Input: part model. Units: mm. Frame: model coordinates. A direction names the side the tool comes from. Round coordinates to 2 decimals unless told otherwise and drop trailing zeros. Loops run counter-clockwise (first coordinate to the right, second up) from the corner with the lowest first, then second, coordinate; pieces in that order, holes last. Notation, with made-up numbers: M 69,44 L 105,44 A26 ccw 105,69 Z; hole C 74.25,5.5 d11. An arc over 180 degrees is marked long. Use one line per item in the form item = value. Start each with the question number.
Q1. Section query B-B, the plane x = 4.5. Output: boundary loops of the cut face in (y, z), and give its area (3 significant figures).
Q2. Ray query, line 1 along Z through (x, y) = (-3, 0.65); line 2 along Z through (x, y) = (13.5, 1); line 3 along X through (y, z) = (0.8, 5.75). Return the intervals inside material, ascending.
Q3. Section query A-A, the plane z = -3. Output: boundary loops of the cut face in (x, y), and give its area (3 significant figures).
Q4. First-contact query: P1, Ø0.9, axis at x = 17.5, y = 0, coming from the +Z side; P2, Ø0.9, axis at x = 17, y = -1, coming from the -Z side. Flat tips, straight axial feed; report the tip coordinate or a pass-through.
Q5. Section query D-D, the plane z = 0. Output: boundary loops of the cut face in (x, y), and give its area (3 significant figures).
Q6. Mould query, pull axis Z, two halves, no side actions, for faces 4 (the flat face through (0, -2.5, 11)), 5 (the cylindrical face through (17.64, -0.04, -11.1)), 6 (the cylindrical face through (-12.64, -0.04, -8.1)). Classes: pulls with the +Z half, pulls with the -Z half, needs draft (parallel to the pull), parting line crosses it, or undercut.
Q7. Section query C-C, the plane y = 1.5. Output: boundary loops of the cut face in (x, z), and give its area (3 significant figures).
Q8. Access query for faces 1 (the flat face through (17, 0, -2)), 2 (the flat face through (1, 0, 9)), 3 (the flat face through (0, 2.5, 11)). Directions: +Z, -Z, +X, -X, +Y, -Y. A direction counts if a zero-diameter tool reaches every point of the face in a straight line with its end or side. Return the directions, or none.
```python
from build123d import *

# Parameters (mm, degrees)
F1_DEPTH = 2.5
F2_R     = 3


with BuildPart() as f1:
    # F0 (on Front) → F1 (new body, symmetric)
    with BuildSketch(Plane.XZ):
        with BuildLine():
            Line((18.5, 12), (-18.5, 12))
            Line((-18.5, 12), (-18.5, -12))
            Line((-18.5, -12), (18.5, -12))
            Line((18.5, -12), (18.5, -2))
            Line((18.5, -2), (15.5, -2))
            Line((15.5, -2), (15.5, -9))
            Line((15.5, -9), (-13.5, -9))
            Line((-13.5, -9), (-13.5, -1.5))
            ThreePointArc((-13.5, -1.5), (-16.714869, 0), (-13.5, 1.5))
            Line((-13.5, 1.5), (-13.5, 9))
            Line((-13.5, 9), (15.5, 9))
            Line((15.5, 9), (15.5, 2))
            Line((15.5, 2), (18.5, 2))
            Line((18.5, 2), (18.5, 12))
        make_face()
    extrude(amount=F1_DEPTH, both=True)

    # F2
    f2_edges = [f1.edges().sort_by_distance(p)[0] for p in [
        (18.5, 0, 12),
        (18.5, 0, -12),
        (-18.5, 0, 12),
        (-18.5, 0, -12),
        (15.5, 0, -9),
        (15.5, 0, 9),
        (-13.5, 0, 9),
        (-13.5, 0, -9),
    ]]
    fillet(f2_edges, radius=F2_R)


solid = f1.part
```
Results found:
q1.outline = M -2.5,-12 L 2.5,-12 L 2.5,-9 L -2.5,-9 Z; M -2.5,9 L 2.5,9 L 2.5,12 L -2.5,12 Z
q1.area = 30.0 mm²
q2.line_1 = -12 to -9, 9 to 12
q2.line_2 = -12 to -8.83, 8.83 to 12
q2.line_3 = -18.5 to -13.5, 15.5 to 18.5
q3.outline = M -18.5,-2.5 L -13.5,-2.5 L -13.5,2.5 L -18.5,2.5 Z; M 15.5,-2.5 L 18.5,-2.5 L 18.5,2.5 L 15.5,2.5 Z
q3.area = 40.0 mm²
q4.P1 = 11.57
q4.P2 = -11.81
q5.outline = M -18.5,-2.5 L -16.71,-2.5 L -16.71,2.5 L -18.5,2.5 Z
q5.area = 8.93 mm²
q6.face_4 = needs draft
q6.face_5 = pulls with the -Z half
q6.face_6 = undercut
q7.outline = M -18.5,-9 A3 ccw -15.5,-12 L 15.5,-12 A3 ccw 18.5,-9 L 18.5,-2 L 15.5,-2 L 15.5,-6 A3 cw 12.5,-9 L -10.5,-9 A3 cw -13.5,-6 L -13.5,-1.5 A1.96 cw long -13.5,1.5 L -13.5,6 A3 cw -10.5,9 L 12.5,9 A3 cw 15.5,6 L 15.5,2 L 18.5,2 L 18.5,9 A3 ccw 15.5,12 L -15.5,12 A3 ccw -18.5,9 Z
q7.area = 343 mm²
q8.face_1 = +X, +Y, -Y
q8.face_2 = +Y, -Y
q8.face_3 = +Z, -Z, +X, -X, +Y
